For this review, take the finished solid that the model builds, in its own axes (mm). Face numbers are marked on the shaded views. A direction names the side the tool comes from. Round coordinates to 2 decimals unless told otherwise and drop trailing zeros. Write each loop counter-clockwise with the first axis right and the second up, starting at its lowest first coordinate (ties: lowest second). Pieces come first, ordered by that corner, then holes. Notation, with made-up numbers: (11.5, 29.25) -> (33.5, 29.25) arc R26 ccw to (33.5, 48.25) -> close; hole circle Ø9 at (-39, 25.5). An arc over 180 degrees is marked (long way). Answer in a Markdown table with one row per item.
from build123d import *

# Parameters (mm, degrees)
BOSS_EXTRUDE1_DEPTH  = 145
M4_CLEARANCE_HOLE1_D = 4.5
HOLE1_D              = 4.5
HOLE1_DEPTH          = 6
SKETCH8_W            = 5
SKETCH8_H            = 145
CUT_EXTRUDE1_DEPTH   = 4


with BuildPart() as part:
    # Sketch1 → Boss-Extrude1 (new body)
    with BuildSketch(Plane(origin=(0, 260, 0), x_dir=(-1, 0, 0), z_dir=(0, -1, 0))):
        Polygon((71.5, -127.5), (61.5, -127.5), (61.5, -97.5), (71.5, -97.5), (71.5, -102.5), (67.5, -102.5), (67.5, -122.5), (71.5, -122.5), align=None)
    extrude(amount=BOSS_EXTRUDE1_DEPTH)

    # M4 Clearance Hole1 (through all)
    with Locations(Plane(origin=(-61.5, 0, 0), x_dir=(0, 0, -1), z_dir=(1, 0, 0))):
        with Locations((-112.5, 247.5), (-112.5, 127.5)):
            Hole(M4_CLEARANCE_HOLE1_D / 2)

    # Hole1
    with Locations(Plane(origin=(-61.5, 0, 0), x_dir=(0, 0, -1), z_dir=(1, 0, 0))):
        with Locations((-104, 216), (-121, 216), (-104, 159), (-121, 159)):
            Hole(HOLE1_D / 2, depth=HOLE1_DEPTH)

    # Sketch8 → Cut-Extrude1 (cut)
    with BuildSketch(Plane.ZY.offset(71.5)):
        with Locations((125, 187.5)):
            Rectangle(SKETCH8_W, SKETCH8_H)
    extrude(amount=-CUT_EXTRUDE1_DEPTH, mode=Mode.SUBTRACT)


solid = part.part
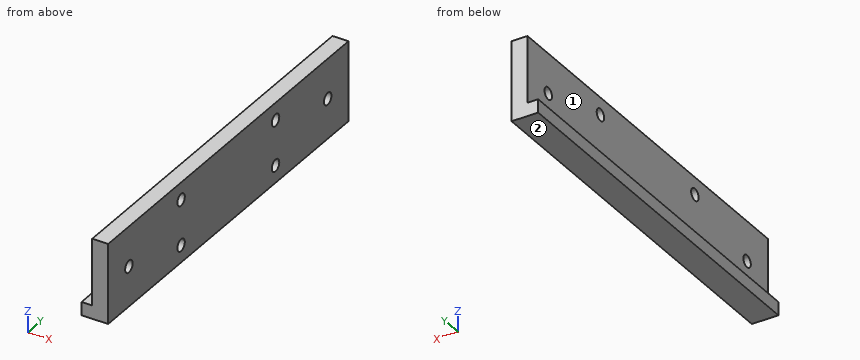
1) Consider section C-C on y = 159. State the section outline as (x, z) points, then the cut area to 3 significant figures.
Solved:
| item | result |
|---|---|
| outline | (-71.5, 97.5) -> (-61.5, 97.5) -> (-61.5, 101.75) -> (-67.5, 101.75) -> (-67.5, 102.5) -> (-71.5, 102.5) -> close; (-67.5, 106.25) -> (-61.5, 106.25) -> (-61.5, 118.75) -> (-67.5, 118.75) -> close; (-67.5, 123.25) -> (-61.5, 123.25) -> (-61.5, 127.5) -> (-67.5, 127.5) -> close |
| area | 146 mm² |
2) Consider section B-B on x = -65. State the section outline as (y, z) points, then the cut area to 3 significant figures.
Solved:
| item | result |
|---|---|
| outline | (115, 97.5) -> (260, 97.5) -> (260, 127.5) -> (115, 127.5) -> close; hole circle Ø4.5 at (127.5, 112.5); hole circle Ø4.5 at (159, 104); hole circle Ø4.5 at (159, 121); hole circle Ø4.5 at (216, 104); hole circle Ø4.5 at (216, 121); hole circle Ø4.5 at (247.5, 112.5) |
| area | 4,250 mm² |
3) For line 1 (Y direction, x = -62.65, z = 112.5); line 2 (Z direction, x = -63.65, y = 216); line 3 (Y direction, x = -63.65, z = 104), list the stretches that pass through material, from the lowest coordinate up. Write a range as [from, to].
Solved:
| item | result |
|---|---|
| line 1 | [115, 125.25], [129.75, 245.25], [249.75, 260] |
| line 2 | [97.5, 101.75], [106.25, 118.75], [123.25, 127.5] |
| line 3 | [115, 156.75], [161.25, 213.75], [218.25, 260] |
4) Consider section D-D on z = 112.5. State the section outline as (x, y) points.
Solved:
| item | result |
|---|---|
| outline | (-67.5, 115) -> (-61.5, 115) -> (-61.5, 125.25) -> (-67.5, 125.25) -> close; (-67.5, 129.75) -> (-61.5, 129.75) -> (-61.5, 245.25) -> (-67.5, 245.25) -> close; (-67.5, 249.75) -> (-61.5, 249.75) -> (-61.5, 260) -> (-67.5, 260) -> close |
5) Consider section A-A on y = 127.5. State the section outline as (x, z) points, then the cut area to 3 significant figures.
Solved:
| item | result |
|---|---|
| outline | (-71.5, 97.5) -> (-61.5, 97.5) -> (-61.5, 110.25) -> (-67.5, 110.25) -> (-67.5, 102.5) -> (-71.5, 102.5) -> close; (-67.5, 114.75) -> (-61.5, 114.75) -> (-61.5, 127.5) -> (-67.5, 127.5) -> close |
| area | 173 mm² |
6) Clearance check with flat-ended pins moving along their axes: pin 1 Ø4 at (y, z) = (216, 104) entering from +X; pin 2 Ø7 at (y, z) = (247.5, 112.5) entering from -X; pin 3 Ø1.2 at (x, y) = (-70.5, 185) entering from +Z. State where each tip first meets the part, or that it passes through.
Solved:
| item | result |
|---|---|
| pin 1 | x = -67.5 |
| pin 2 | x = -67.5 |
| pin 3 | z = 102.5 |
7) For the marked faces 1 and 2, list the 3-axis set-ups (+Z, -Z, +X, -X, +Y, -Y) from which the entire face can be reached by the end or side of a thin tool; tool diameter is ignored.
Solved:
| item | result |
|---|---|
| face 1 | +Z, -X, +Y, -Y |
| face 2 | -Z, +X, -X, +Y, -Y |
